Part model, mm, in its own coordinate system. A direction names the side the tool comes from. Coordinates: 2 decimals unless noted, no trailing zeros. Loops run counter-clockwise (first coordinate to the right, second up) from the corner with the lowest first, then second, coordinate; pieces in that order, holes last. Notation, with made-up numbers: (-5.75, 72.5) - (36.25, 72.5) arc R22 cw to (36.25, 99.5) - close; hole circle Ø7 at (-0.75, 88). An arc over 180 degrees is marked (long way). Use a Markdown table: item, result. Add a question column.
1. Band-saw the part on A-A, the plane x = 0. Give the cut face in (y, z), plus the area to 3 significant figures.
2. Pull direction Z, two halves, no side cores. Call faces 3 (the flat face through (-1.1, 12.5, -0.15)), 4 (the cylindrical face through (2.44, 6.41, 0.54)), 5 (the flat face through (1, 13, -1)): pulls with the +Z half, pulls with the -Z half, needs draft (parallel to the pull), parting line crosses it, or undercut.
3. Band-saw the part on C-C, the plane y = 6. Give the cut face in (x, z).
4. Wall check: probe 1 along Y at (x, z) = (0.05, 0.45); probe 2 along Z at (x, y) = (0.1, 2.25); probe 3 along Z at (x, y) = (-2.1, 6.5). Give the ranges that are in metal, low to high. Write a range as [from, to].
5. 3-axis set-ups, long thin cutter, end or side, ignore diameter. For faces 1 (the flat face through (0.15, 12.5, 1.1)), 2 (the flat face through (0, 0, 0)): which of +Z, -Z, +X, -X, +Y, -Y reach the whole face in a straight line?
6. Band-saw the part on B-B, the plane z = 1.5. Give the cut face in (x, y).
7. Drop flat-ended pins along their axis: pin 1 (0.8 mm diameter, centred on y = 12.5, z = -1.5, fed in from +X) (3 decimals); pin 2 (1.5 mm diameter, centred on y = 9, z = 1, fed in from +X); pin 3 (1.1 mm diameter, centred on y = 12.5, z = -1, fed in from -X). Give the stop position or say it passes through.
from build123d import *

# Parameters (mm, degrees)
SKETCH2_R           = 2.5
BOSS_EXTRUDE1_DEPTH = 13
SKETCH3_W           = 1.85
SKETCH3_H           = 0.3
SKETCH3_W_2         = 0.3
SKETCH3_H_2         = 1.85
CUT_EXTRUDE1_DEPTH  = 1


with BuildPart() as part:
    # Sketch2 → Boss-Extrude1 (new body)
    with BuildSketch(Plane(origin=(0, 0, 0), x_dir=(1, 0, 0), z_dir=(0, 1, 0))):
        with Locations(Location((0, 0, 0), (0, 0, 90))):
            Circle(SKETCH2_R)
    extrude(amount=BOSS_EXTRUDE1_DEPTH)

    # Sketch3 → Cut-Extrude1 (cut)
    with BuildSketch(Plane(origin=(0, 13, 0), x_dir=(1, 0, 0), z_dir=(0, 1, 0))):
        with Locations((1.075, 0)):
            Rectangle(SKETCH3_W, SKETCH3_H)
        Rectangle(SKETCH3_W_2, SKETCH3_H)
        with Locations((-1.075, 0)):
            Rectangle(SKETCH3_W, SKETCH3_H)
        with Locations((0, 1.075)):
            Rectangle(SKETCH3_W_2, SKETCH3_H_2)
        with Locations((0, -1.075)):
            Rectangle(SKETCH3_W_2, SKETCH3_H_2)
    extrude(amount=-CUT_EXTRUDE1_DEPTH, mode=Mode.SUBTRACT)


solid = part.part
Geometry check:
| question | item | result |
|---|---|---|
| 1 | outline | (0, -2.5) - (13, -2.5) - (13, -2) - (12, -2) - (12, 2) - (13, 2) - (13, 2.5) - (0, 2.5) - close |
| 1 | area | 61.0 mm^2 |
| 2 | face 3 | undercut |
| 2 | face 4 | parting line crosses it |
| 2 | face 5 | needs draft |
| 3 | outline | circle Ø5 at (0, 0) |
| 4 | probe 1 | y = [0, 12] |
| 4 | probe 2 | z = [-2.5, 2.5] |
| 4 | probe 3 | z = [-1.36, 1.36] |
| 5 | face 1 | +Y |
| 5 | face 2 | +Z, -Z, +X, -X, -Y |
| 6 | outline | (-2, 0) - (2, 0) - (2, 13) - (0.15, 13) - (0.15, 12) - (-0.15, 12) - (-0.15, 13) - (-2, 13) - close |
| 7 | pin 1 | stops at x = 2.245 |
| 7 | pin 2 | stops at x = 2.49 |
| 7 | pin 3 | stops at x = -2.46 |
